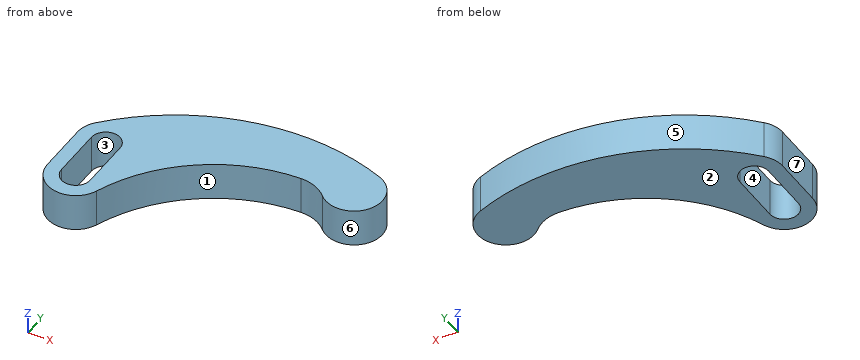
from build123d import *

# Parameters (mm, degrees)
BOSS_EXTRUDE1_DEPTH = 25.4


with BuildPart() as part:
    # Sketch1 → Boss-Extrude1 (new body)
    with BuildSketch(Plane.XY):
        with BuildLine():
            Line((-165.1, -69.596), (-165.1, -35.56))
            ThreePointArc((-165.1, -35.56), (-163.834131861, -28.731592137), (-160.20476074, -22.810676552))
            ThreePointArc((-160.20476074, -22.810676552), (-83.019510627, 23.268882931), (6.709524974, 17.829323448))
            ThreePointArc((6.709524974, 17.829323448), (16.063246399, -10.240830783), (-13.332222743, -13.607142857))
            ThreePointArc((-13.332222743, -13.607142857), (-21.95402191, -8.057064985), (-32.067687872, -6.368116766))
            ThreePointArc((-32.067687872, -6.368116766), (-90.731121166, -26.656656194), (-128.169572983, -76.168125204))
            ThreePointArc((-128.169572983, -76.168125204), (-149.387691218, -88.351327705), (-165.1, -69.596))
        make_face()
        with BuildLine():
            Line((-155.702, -35.56), (-155.702, -69.596))
            ThreePointArc((-155.702, -69.596), (-146.05, -79.248), (-136.398, -69.596))
            Line((-136.398, -69.596), (-136.398, -35.56))
            ThreePointArc((-136.398, -35.56), (-146.05, -25.908), (-155.702, -35.56))
        make_face(mode=Mode.SUBTRACT)
    extrude(amount=BOSS_EXTRUDE1_DEPTH)


solid = part.part
Check sheet for the modelled part. Datum: model origin and axes. Units: mm. Face numbers are marked on the shaded views. A direction names the side the tool comes from. Round coordinates to 2 decimals unless told otherwise and drop trailing zeros. Order: outer loops, then holes, each group sorted by start corner. A loop starts at its lowest first (then second) coordinate and runs counter-clockwise, first axis right, second up.
Q1. Set-up check for the marked faces 1, 2 and 3: record each of +Z, -Z, +X, -X, +Y, -Y from which the full face is reachable in a straight line by a thin tool's end or side.
Filled sheet:
face 1: +Z, -Z, -Y
face 2: -Z, +X, -X, +Y, -Y
face 3: +Z, -Z
Q2. Cross-section at D-D, the plane y = 0. Enter the section's corners in (x, z), plus the area to 3 significant figures.
Filled sheet:
outline: (-134.43, 0) - (19.05, 0) - (19.05, 25.4) - (-134.43, 25.4) - close
area: 3,900 mm2
Q3. Cross-section at A-A, the plane z = 15.25. Enter the section's corners in (x, y), plus the area to 3 significant figures.
Filled sheet:
outline: (-165.1, -69.6) arc R19.05 ccw to (-128.17, -76.17) arc R106.68 cw to (-32.07, -6.37) arc R25.4 cw to (-13.33, -13.61) arc R19.05 ccw (long way) to (6.71, 17.83) arc R152.4 ccw to (-160.2, -22.81) arc R19.05 ccw to (-165.1, -35.56) - close; hole (-155.7, -69.6) arc R9.65 ccw to (-136.4, -69.6) - (-136.4, -35.56) arc R9.65 ccw to (-155.7, -35.56) - close
area: 8,080 mm2
Q4. Scan lines: L1, parallel to X at y = -41, z = 8.25; L2, parallel to X at y = -63, z = 14.25; L3, parallel to Y at x = -146, z = 6.75. Record each from-to range of solid material in increasing order.
Filled sheet:
L1: x = -165.1 to -155.7, -136.4 to -106.78
L2: x = -165.1 to -155.7, -136.4 to -122.29
L3: y = -88.65 to -79.25, -25.91 to -8.97
Q5. Depth check by flat-ended pin: P1, Ø7.5, axis at y = -54.5, z = 13.5, coming from the +X side; P2, Ø6, axis at x = -16, y = 13.5, coming from the -Z side; P3, Ø1, axis at x = -27.5, z = 18.5, coming from the +Y side; P4, Ø2, axis at x = -72.5, z = 18.5, coming from the +Y side. Enter the tip coordinate at first touch or a pass-through.
Filled sheet:
P1: stops at x = -114.69
P2: stops at z = 0
P3: stops at y = 26.41
P4: stops at y = 25.61
Q6. Cross-section at C-C, the plane x = -146.05. Enter the section's corners in (y, z).
Filled sheet:
outline: (-88.65, 0) - (-79.25, 0) - (-79.25, 25.4) - (-88.65, 25.4) - close; (-25.91, 0) - (-9.01, 0) - (-9.01, 25.4) - (-25.91, 25.4) - close
Q7. Cross-section at B-B, the plane y = -48.5. Enter the section's corners in (x, z).
Filled sheet:
outline: (-165.1, 0) - (-155.7, 0) - (-155.7, 25.4) - (-165.1, 25.4) - close; (-136.4, 0) - (-113.03, 0) - (-113.03, 25.4) - (-136.4, 25.4) - close
Q8. Draft check along Y on the marked faces 4, 5, 6 and 7. Enter one of: pulls with the +Y half, pulls with the -Y half, needs draft (parallel to the pull), parting line crosses it, or undercut.
Filled sheet:
face 4: undercut
face 5: pulls with the +Y half
face 6: parting line crosses it
face 7: needs draft
